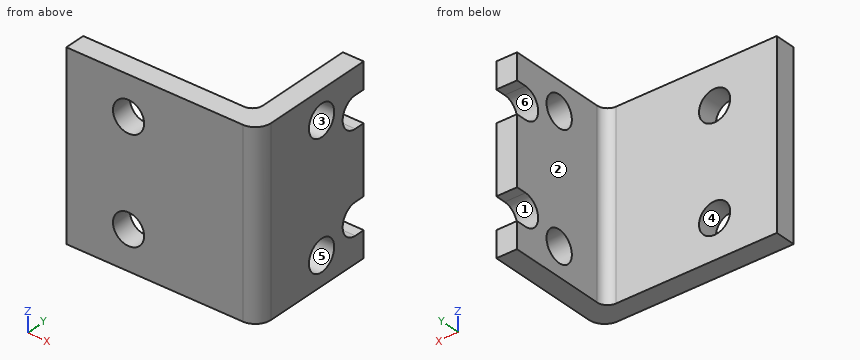
```python
from build123d import *

# Parameters (mm, degrees)
EXTRUDE_1_DEPTH     = 35
SKETCH_2_R          = 3
CUT_EXTRUDE_2_DEPTH = 35
SKETCH_3_R          = 3
EXTRUDE_4_DEPTH     = 37
SKETCH_3_2_R        = 3
CUT_EXTRUDE_5_DEPTH = 57.771215716


with BuildPart() as part:
    # 草图1 → 拉伸1 (new body)
    with BuildSketch(Plane.XY):
        with BuildLine():
            ThreePointArc((18.167628925, -21.079292929), (19.581842488, -20.493506492), (20.167628925, -19.079292929))
            Line((20.167628925, -19.079292929), (20.167628925, -0.079292929))
            Line((20.167628925, -0.079292929), (24.167628925, -0.079292929))
            Line((24.167628925, -0.079292929), (24.167628925, -22.079292929))
            ThreePointArc((24.167628925, -22.079292929), (23.288949269, -24.200613273), (21.167628925, -25.079292929))
            Line((21.167628925, -25.079292929), (-12.832371075, -25.079292929))
            Line((-12.832371075, -25.079292929), (-12.832371075, -21.079292929))
            Line((-12.832371075, -21.079292929), (18.167628925, -21.079292929))
        make_face()
    extrude(amount=EXTRUDE_1_DEPTH)

    # 草图2 → 拉伸2 (cut)
    with BuildSketch(Plane.XZ.offset(25.079292929)):
        with Locations((-0.832371075, 7.5)):
            Circle(SKETCH_2_R)
        with Locations((-0.832371075, 27.5)):
            Circle(SKETCH_2_R)
    extrude(amount=-CUT_EXTRUDE_2_DEPTH, mode=Mode.SUBTRACT)

    # 草图3 → 拉伸4 (add, through all)
    with BuildSketch(Plane(origin=(24.167628925, 0, 0), x_dir=(0, 0, -1), z_dir=(1, 0, 0))):
        with Locations(Location((-5.5, -10.079292929, 0), (0, 0, 90))):
            Circle(SKETCH_3_R)
        with Locations(Location((-29.5, -10.079292929, 0), (0, 0, 90))):
            Circle(SKETCH_3_R)
        with BuildLine():
            Line((-5, -2.079292929), (-5, 0.455458984))
            Line((-5, 0.455458984), (-11, 0.455458984))
            Line((-11, 0.455458984), (-11, -2.079292929))
            ThreePointArc((-11, -2.079292929), (-8, -5.079292929), (-5, -2.079292929))
        make_face()
        with BuildLine():
            Line((-24, -2.079292929), (-24, 0.455458984))
            Line((-24, 0.455458984), (-30, 0.455458984))
            Line((-30, 0.455458984), (-30, -2.079292929))
            ThreePointArc((-30, -2.079292929), (-27, -5.079292929), (-24, -2.079292929))
        make_face()
    extrude(amount=-EXTRUDE_4_DEPTH)

    # 草图3<2> → 拉伸5 (cut, through all)
    with BuildSketch(Plane(origin=(24.167628925, 0, 0), x_dir=(0, 0, -1), z_dir=(1, 0, 0))):
        with Locations(Location((-5.5, -10.079292929, 0), (0, 0, 90))):
            Circle(SKETCH_3_2_R)
        with Locations(Location((-29.5, -10.079292929, 0), (0, 0, 90))):
            Circle(SKETCH_3_2_R)
        with BuildLine():
            Line((-5, -2.079292929), (-5, 0.455458984))
            Line((-5, 0.455458984), (-11, 0.455458984))
            Line((-11, 0.455458984), (-11, -2.079292929))
            ThreePointArc((-11, -2.079292929), (-8, -5.079292929), (-5, -2.079292929))
        make_face()
        with BuildLine():
            Line((-24, -2.079292929), (-24, 0.455458984))
            Line((-24, 0.455458984), (-30, 0.455458984))
            Line((-30, 0.455458984), (-30, -2.079292929))
            ThreePointArc((-30, -2.079292929), (-27, -5.079292929), (-24, -2.079292929))
        make_face()
    extrude(amount=-CUT_EXTRUDE_5_DEPTH, mode=Mode.SUBTRACT)


solid = part.part
```
Work out the finished part from the listing and answer in its coordinate system (mm). Face numbers are marked on the shaded views. A direction names the side the tool comes from. Round coordinates to 2 decimals unless told otherwise and drop trailing zeros. Order: outer loops, then holes, each group sorted by start corner. A loop starts at its lowest first (then second) coordinate and runs counter-clockwise, first axis right, second up.
Q1. A tool of negligible diameter and unlimited length cuts with its end or side. For the marked faces 1 and 2, from which of +Z, -Z, +X, -X, +Y, -Y can it reach the whole face along a straight path? Write none if from no direction.
Solution:
face 1: +X, -X, +Y
face 2: +Z, -Z, -X, +Y
Q2. A cutting plane is placed at A-A, the plane z = 3.5. Determine the outline of the cut face in (x, y), then the cut area to 3 significant figures.
Solution:
outline: (-12.83, -25.08) - (21.17, -25.08) arc R3 ccw to (24.17, -22.08) - (24.17, -12.32) - (20.17, -12.32) - (20.17, -19.08) arc R2 cw to (18.17, -21.08) - (-12.83, -21.08) - close; (20.17, -7.84) - (24.17, -7.84) - (24.17, -0.08) - (20.17, -0.08) - close
area: 213 mm2
Q3. The mould has two halves that part along Y. Classify the marked faces 3, 4, 5 and 6: pulls with the +Y half, pulls with the -Y half, needs draft (parallel to the pull), parting line crosses it, or undercut.
Solution:
face 3: undercut
face 4: needs draft
face 5: undercut
face 6: pulls with the +Y half
Q4. Given pin 1 Ø3.5 at (x, z) = (-0.83, 7.5) entering from +Y; pin 2 Ø9.5 at (y, z) = (-10.08, 5.5) entering from -X; pin 3 Ø12 at (x, z) = (-6.5, 4) entering from +Y, each flat-ended and moving along its own axis, determine where each tip first touches the part or whether it passes through.
Solution:
pin 1: passes through
pin 2: stops at x = 20.17
pin 3: stops at y = -21.08
Q5. A cutting plane is placed at B-B, the plane y = -9. Determine the outline of the cut face in (x, z), then the cut area to 3 significant figures.
Solution:
outline: (20.17, 0) - (24.17, 0) - (24.17, 2.7) - (20.17, 2.7) - close; (20.17, 8.3) - (24.17, 8.3) - (24.17, 26.7) - (20.17, 26.7) - close; (20.17, 32.3) - (24.17, 32.3) - (24.17, 35) - (20.17, 35) - close
area: 95.2 mm2
Q6. A cutting plane is placed at D-D, the plane y = -23. Determine the outline of the cut face in (x, z).
Solution:
outline: (-12.83, 0) - (24.02, 0) - (24.02, 35) - (-12.83, 35) - close; hole circle Ø6 at (-0.83, 7.5); hole circle Ø6 at (-0.83, 27.5)
Q7. A cutting plane is placed at C-C, the plane z = 8. Determine the outline of the cut face in (x, y).
Solution:
outline: (-12.83, -25.08) - (-3.79, -25.08) - (-3.79, -21.08) - (-12.83, -21.08) - close; (2.13, -25.08) - (21.17, -25.08) arc R3 ccw to (24.17, -22.08) - (24.17, -11.74) - (20.17, -11.74) - (20.17, -19.08) arc R2 cw to (18.17, -21.08) - (2.13, -21.08) - close; (20.17, -8.42) - (24.17, -8.42) - (24.17, -5.08) - (20.17, -5.08) - close
Q8. Find the intervals of material crossed by line 1 along Y through (x, z) = (13.5, 4.5); line 2 along X through (y, z) = (-9.5, 24.5); line 3 along Y through (x, z) = (22, 29), in increasing order.
Solution:
line 1: y = -25.08 to -21.08
line 2: x = 20.17 to 24.17
line 3: y = -24.96 to -13.04, -7.12 to -4.32
